Can you work these out from the drawing? Everything is in mm from the part's minimum corner. Round coordinates to 2 decimals unless told otherwise and drop trailing zeros. Write each loop counter-clockwise with the first axis right and the second up, starting at its lowest first coordinate (ties: lowest second). Pieces come first, ordered by that corner, then holes. Notation, with made-up numbers: M -7.75,28 L 6.25,28 A18 cw 6.25,55 Z; hole C 43,52.5 d3. An arc over 180 degrees is marked long. Use a Markdown table: item, result. Add a question column.
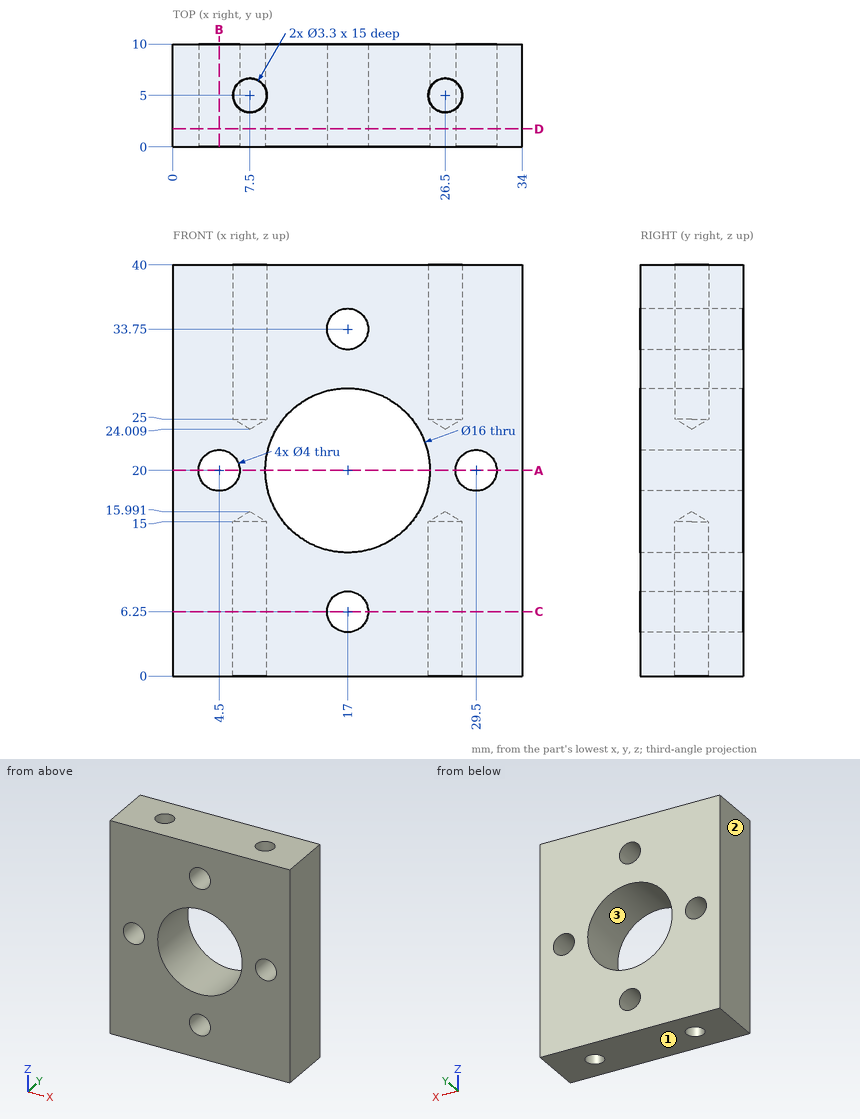
Item 1: For pin 1 Ø2 at (x, y) = (26.5, 5) entering from +Z; pin 2 Ø2.5 at (x, z) = (29.5, 20) entering from +Y, each with a flat end and sliding along its axis, tell me the tip position at first contact or that it passes through.
Item 2: I need wall thicknesses on probe 1 along X at (y, z) = (5, 33.75); probe 2 along X at (y, z) = (7.5, 33.75); probe 3 along Z at (x, y) = (18, 6.75). Which ranges of each line are inside material? Lowest first, please. Write a range as from..to.
Item 3: Imagine slicing it at B-B on x = 4.5. List the corners of the cut face in (y, z) for me.
Item 4: Imagine slicing it at D-D on y = 1.75. List the corners of the cut face in (x, z) for me.
Item 5: Imagine slicing it at A-A on z = 20. List the corners of the cut face in (x, y) for me, plus the area to 3 significant figures.
Item 6: Imagine slicing it at C-C on z = 6.25. List the corners of the cut face in (x, y) for me, plus the area to 3 significant figures.
Item 7: If we mould it in two halves opening along X, with no side actions, what happens to the marked faces 1, 2 and 3? For each: +X half, -X half, draft (parallel to the pull), parting line (faces both ways), or undercut.
The answers:
| question | item | result |
|---|---|---|
| 1 | pin 1 | z = 24.61 |
| 1 | pin 2 | through |
| 2 | probe 1 | 0..5.85, 9.15..15, 19..24.85, 28.15..34 |
| 2 | probe 2 | 0..15, 19..34 |
| 2 | probe 3 | 0..4.52, 7.98..12.06, 27.94..32.02, 35.48..40 |
| 3 | outline | M 0,0 L 10,0 L 10,18 L 0,18 Z; M 0,22 L 10,22 L 10,40 L 0,40 Z |
| 4 | outline | M 0,0 L 34,0 L 34,40 L 0,40 Z; hole C 4.5,20 d4; hole C 17,20 d16; hole C 17,6.25 d4; hole C 17,33.75 d4; hole C 29.5,20 d4 |
| 5 | outline | M 0,0 L 2.5,0 L 2.5,10 L 0,10 Z; M 6.5,0 L 9,0 L 9,10 L 6.5,10 Z; M 25,0 L 27.5,0 L 27.5,10 L 25,10 Z; M 31.5,0 L 34,0 L 34,10 L 31.5,10 Z |
| 5 | area | 100 mm² |
| 6 | outline | M 0,0 L 15,0 L 15,10 L 0,10 Z; M 19,0 L 34,0 L 34,10 L 19,10 Z; hole C 7.5,5 d3.3; hole C 26.5,5 d3.3 |
| 6 | area | 283 mm² |
| 7 | face 1 | draft |
| 7 | face 2 | -X half |
| 7 | face 3 | undercut |
